Geometry: final body of the model. Coordinates: model frame, mm. A direction names the side the tool comes from. Give positions to 0.01 mm unless a question says otherwise; leave off trailing zeros. Write each loop counter-clockwise with the first axis right and the second up, starting at its lowest first coordinate (ties: lowest second). Pieces come first, ordered by that corner, then holes.
from build123d import *

# Parameters (mm, degrees)
ESQUISSE1_W             = 15
ESQUISSE1_H             = 24.52
BOSS_EXTRU_1_DEPTH      = 20.5
ENL_V_MAT_EXTRU_2_DEPTH = 3
ENL_V_START             = -3
ENL_V_MAT_EXTRU_1_DEPTH = 3
CHANFREIN2_SIZE         = 4
CHANFREIN2_SIZE_2       = 25.255006059
CHANFREIN3_SIZE         = 24.820002444
CHANFREIN3_SIZE_2       = 0.78


with BuildPart() as part:
    # Esquisse1 → Boss.-Extru.1 (new body)
    with BuildSketch(Plane.XY):
        with Locations((-7.5, 12.26)):
            Rectangle(ESQUISSE1_W, ESQUISSE1_H)
    extrude(amount=-BOSS_EXTRU_1_DEPTH)

    # Esquisse3 → Enlèv. mat.-Extru.2 (cut)
    with BuildSketch(Plane.XZ):
        with BuildLine():
            ThreePointArc((-5.5, -15.375), (-6.085786438, -13.960786438), (-7.5, -13.375))
            Line((-7.5, -13.375), (-7.5, -15.375))
            Line((-7.5, -15.375), (-7.5, -17.375))
            ThreePointArc((-7.5, -17.375), (-6.085786438, -16.789213562), (-5.5, -15.375))
        make_face()
        with BuildLine():
            Line((-7.5, -15.375), (-7.5, -13.375))
            ThreePointArc((-7.5, -13.375), (-9.5, -15.375), (-7.5, -17.375))
            Line((-7.5, -17.375), (-7.5, -15.375))
        make_face()
        with BuildLine():
            ThreePointArc((-7.5, -5.6875), (-9.5, -7.6875), (-7.5, -9.6875))
            Line((-7.5, -9.6875), (-7.5, -5.6875))
        make_face()
        with BuildLine():
            Line((-7.5, -5.6875), (-7.5, -9.6875))
            ThreePointArc((-7.5, -9.6875), (-6.085786438, -9.101713562), (-5.5, -7.6875))
            ThreePointArc((-5.5, -7.6875), (-6.085786438, -6.273286438), (-7.5, -5.6875))
        make_face()
    extrude(amount=-ENL_V_MAT_EXTRU_2_DEPTH, mode=Mode.SUBTRACT)

    # Esquisse2 → Enlèv. mat.-Extru.1 (cut)
    with BuildSketch(Plane(origin=(0, 24.52, 0), x_dir=(1, 0, 0), z_dir=(0, 1, 0)).offset(ENL_V_START)):
        with BuildLine():
            ThreePointArc((-7.5, 17.375), (-9.5, 15.375), (-7.5, 13.375))
            Line((-7.5, 13.375), (-7.5, 17.375))
        make_face()
        with BuildLine():
            Line((-7.5, 17.375), (-7.5, 13.375))
            ThreePointArc((-7.5, 13.375), (-6.085786438, 13.960786438), (-5.5, 15.375))
            ThreePointArc((-5.5, 15.375), (-6.085786438, 16.789213562), (-7.5, 17.375))
        make_face()
        with BuildLine():
            ThreePointArc((-5.5, 5.125), (-6.085786438, 6.539213562), (-7.5, 7.125))
            Line((-7.5, 7.125), (-7.5, 3.125))
            ThreePointArc((-7.5, 3.125), (-6.085786438, 3.710786438), (-5.5, 5.125))
        make_face()
        with BuildLine():
            Line((-7.5, 3.125), (-7.5, 7.125))
            ThreePointArc((-7.5, 7.125), (-9.5, 5.125), (-7.5, 3.125))
        make_face()
    extrude(amount=ENL_V_MAT_EXTRU_1_DEPTH, mode=Mode.SUBTRACT)

    # Chanfrein2
    # the kernel refuses this chamfer: 25.255006059, 4 mm, written as the material it takes off along each edge
    with BuildSketch(Plane(origin=(65.633111729, 0, 0), x_dir=(0, -0.2333366369919624, -0.9723960169793381), z_dir=(-1, 0, 0))) as chanfrein2_piece_1:
        Polygon((CHANFREIN2_SIZE * 0.972396016979, -CHANFREIN2_SIZE * 0.233336636992), (-CHANFREIN2_SIZE_2 * 0.233336636989, -CHANFREIN2_SIZE_2 * 0.972396016968), (0, 0), align=None)
    extrude(amount=146.266223457, mode=Mode.SUBTRACT)

    # Chanfrein3
    # the kernel refuses this chamfer: 24.820002444, 0.78 mm, written as the material it takes off along each edge
    with BuildSketch(Plane(origin=(-79.530828731, 24.52, -20.5), x_dir=(0, -0.999999270212902, -0.0012081281651260673), z_dir=(1, 0, 0))) as chanfrein3_piece_1:
        Polygon((CHANFREIN3_SIZE * 0.999999270211, -CHANFREIN3_SIZE * 0.00120812816512), (-CHANFREIN3_SIZE_2 * 0.00120812816513, -CHANFREIN3_SIZE_2 * 0.999999270213), (0, 0), align=None)
    extrude(amount=144.061657461, mode=Mode.SUBTRACT)


solid = part.part
Q1. Ray query, line 1 along Z through (x, y) = (-7, 2); line 2 along Z through (x, y) = (-2.5, 20); line 3 along Z through (x, y) = (-9.5, 6.5). Return the intervals inside material, ascending.
Filled sheet:
line 1: z = -20.43 to -17.31, -13.44 to -9.62, -5.75 to -3.68
line 2: z = -19.86 to -0.83
line 3: z = -20.29 to -2.97
Q2. Section D-D on z = -16.25. Output: boundary loops of the cut face in (x, y).
Filled sheet:
outline: (-15, 0) - (-9.3, 0) - (-9.3, 3) - (-5.7, 3) - (-5.7, 0) - (0, 0) - (0, 24.52) - (-5.7, 24.52) - (-5.7, 21.52) - (-9.3, 21.52) - (-9.3, 24.52) - (-15, 24.52) - close
Q3. Pin query (flat end, axial travel): P1, Ø2, axis at x = -3, y = 3, coming from the +Z side; P2, Ø4, axis at x = -5.5, y = 3.5, coming from the -Z side; P3, Ø1.2, axis at x = -7.5, z = -15.5, coming from the +Y side. Return the tip coordinate at first contact, or that it passes through.
Filled sheet:
P1: stops at z = -3.37
P2: stops at z = -20.44
P3: stops at y = 21.52
Q4. Section B-B on x = -1.5. Output: boundary loops of the cut face in (y, z), plus the area to 3 significant figures.
Filled sheet:
outline: (0, -20.49) - (24.52, -19.72) - (24.52, -0.12) - (0, -4) - close
area: 443 mm2
Q5. Section C-C on y = 6.5. Output: boundary loops of the cut face in (x, z).
Filled sheet:
outline: (-15, -20.29) - (0, -20.29) - (0, -2.97) - (-15, -2.97) - close
Q6. Section A-A on z = -8.75. Output: boundary loops of the cut face in (x, y).
Filled sheet:
outline: (-15, 0) - (-9.19, 0) - (-9.19, 3) - (-5.81, 3) - (-5.81, 0) - (0, 0) - (0, 24.52) - (-15, 24.52) - close
Q7. Pull-direction query (Z, two-part tool) for faces 1 (the flat face through (-8, 3, -15)), 2 (the flat face through (-7.395, 12.088, -2.085)), 3 (the flat face through (0, 12, -10)); classes: released by +Z, released by -Z, zero draft, split by the parting line, or undercut.
Filled sheet:
face 1: undercut
face 2: released by +Z
face 3: zero draft
Q8. Access query for faces 4 (the flat face through (-8, 24.52, -10)), 5 (the flat face through (-8, 3, -8)), 6 (the flat face through (-8, 21.52, -5)). Directions: +Z, -Z, +X, -X, +Y, -Y. A direction counts if a zero-diameter tool reaches every point of the face in a straight line with its end or side. Return the directions, or none.
Filled sheet:
face 4: +Z, -Z, +X, -X, +Y
face 5: -Y
face 6: +Y
